Autodesk Inventor part; units mm, degrees
ref_plane "YZ Plane" through (0, 0, 0) normal (1, 0, 0) x (0, 1, 0)
ref_plane "XZ Plane" through (0, 0, 0) normal (0, 1, 0) x (-1, 0, 0)
ref_plane "XY Plane" through (0, 0, 0) normal (0, 0, 1) x (1, 0, 0)
sketch "Sketch1" plane through (0, 0, 0) normal (0, 1, 0) x (-1, 0, 0)
  line L0 (29, 0) -> (29, -12)
  line L1 (27, -14) -> (16, -14)
  line L2 (-16, -14) -> (-27, -14)
  line L3 (-29, -12) -> (-29, 12)
  line L4 (-27, 14) -> (-16, 14)
  line L5 (16, 14) -> (27, 14)
  line L6 (29, 12) -> (29, 0)
  line L7 (14, -16) -> (14, -40)
  line L8 (12, -42) -> (-12, -42)
  line L9 (-14, -40) -> (-14, -16)
  line L10 (-14, 16) -> (-14, 40)
  line L11 (-12, 42) -> (12, 42)
  line L12 (14, 40) -> (14, 16)
  arc A0 (29, 12) -> (27, 14) centre (27, 12) ccw
  arc A1 (27, -14) -> (29, -12) centre (27, -12) ccw
  arc A2 (16, -14) -> (14, -16) centre (16, -16) ccw
  arc A3 (12, -42) -> (14, -40) centre (12, -40) ccw
  arc A4 (-14, -40) -> (-12, -42) centre (-12, -40) ccw
  arc A5 (-14, -16) -> (-16, -14) centre (-16, -16) ccw
  arc A6 (-29, -12) -> (-27, -14) centre (-27, -12) ccw
  arc A7 (-27, 14) -> (-29, 12) centre (-27, 12) ccw
  arc A8 (-16, 14) -> (-14, 16) centre (-16, 16) ccw
  arc A9 (-12, 42) -> (-14, 40) centre (-12, 40) ccw
  arc A10 (14, 40) -> (12, 42) centre (12, 40) ccw
  arc A11 (14, 16) -> (16, 14) centre (16, 16) ccw
  point P0 (0, 0)
  point P1 (29, -14)
  point P2 (14, -14)
  point P3 (-14, -14)
  point P4 (-29, -14)
  point P5 (-29, 14)
  point P6 (-14, 14)
  point P7 (14, -42)
  point P8 (-14, 42)
  point P9 (14, 42)
  dimension "d2" = 14
  dimension "d4" = 15
  dimension "d5" = 28
  dimension "d7" = 28
  dimension "d8" = 28
  dimension "d12" = 2
extrude "Extrusion1" add sketch "Sketch1" along normal blind 1
sketch "Sketch2" plane through (0, 1, 0) normal (0, 1, 0) x (1, 0, 0)
  circle A0 centre (0, 0) radius 19
  dimension "d15" = 38
extrude "Extrusion2" add sketch "Sketch2" along normal blind 10
sketch "Sketch3" plane through (0, 11, 0) normal (0, 1, 0) x (1, 0, 0)
  circle A0 centre (0, 0) radius 8
  dimension "d18" = 16
extrude "Extrusion3" add sketch "Sketch3" along normal blind 7
sketch "Sketch4" plane through (0, 18, 0) normal (0, 1, 0) x (1, 0, 0)
  circle A0 centre (0, 0) radius 13.5
  dimension "d21" = 27
extrude "Extrusion4" add sketch "Sketch4" along normal blind 40
sketch "Sketch5" plane through (0, 58, 0) normal (0, 1, 0) x (1, 0, 0)
  line L0 (0, 41.9572) -> (12, 41.9572)
  line L1 (14, 39.9572) -> (14, -40)
  line L2 (12, -42) -> (-12, -42)
  line L3 (-14, -40) -> (-14, 39.9572)
  line L4 (-12, 41.9572) -> (0, 41.9572)
  arc A0 (-12, 41.9572) -> (-14, 39.9572) centre (-12, 39.9572) ccw
  arc A1 (14, 39.9572) -> (12, 41.9572) centre (12, 39.9572) ccw
  arc A2 (12, -42) -> (14, -40) centre (12, -40) ccw
  arc A3 (-14, -40) -> (-12, -42) centre (-12, -40) ccw
  point P0 (0, 0)
  point P1 (-14, 41.9572)
  dimension "d24" = 2
extrude "Extrusion5" add sketch "Sketch5" along normal blind 1
sketch "Sketch6" plane through (0, 1, 0) normal (0, 1, 0) x (1, 0, 0)
  line L0 (0, 0) -> (0, 36)
  line L1 (0, 0) -> (0, -36)
  circle A0 centre (0, 36) radius 2.5
  circle A1 centre (0, -36) radius 2.5
  dimension "d27" = 36
  dimension "d28" = 36
  dimension "d29" = 5
  dimension "d30" = 5
extrude "Extrusion6" add sketch "Sketch6" along normal blind 58
sketch "Sketch7" plane through (0, 0, 0) normal (0, -1, 0) x (1, 0, 0)
  circle A0 centre (0, 0) radius 15
  dimension "d33" = 30
extrude "Extrusion7" add sketch "Sketch7" along normal blind 32
sketch "Sketch8" plane through (0, -32, 0) normal (0, -1, 0) x (1, 0, 0)
  circle A0 centre (0, 0) radius 8
  dimension "d36" = 16
extrude "Extrusion8" add sketch "Sketch8" along normal blind 43
fillet "Fillet1" radius 5 1 edges at (-15, -32, 0)
sketch "Sketch9" plane through (0, -75, 0) normal (0, -1, 0) x (1, 0, 0)
  circle A0 centre (0, 0) radius 4
  circle A1 centre (0, 0) radius 12.3979
  dimension "d40" = 8
extrude "Extrusion9" cut sketch "Sketch9" against normal blind 20
fillet "Fillet2" radius 5 1 edges at (-4, -55, 0)
sketch "Sketch10" plane through (14, 0, 40) normal (1, 0, 0) x (0, 0, -1)
  line L0 (36, -75) -> (44, -75)
  line L1 (36, -75) -> (38.5, -75)
  line L2 (38.5, -75) -> (38.5, -71.9713)
  line L3 (38.5, -71.9713) -> (36, -71.9713)
  line L4 (36, -71.9713) -> (36, -75)
  line L5 (44, -59.899) -> (44, -75)
  line L6 (44, -75) -> (41.5, -75)
  line L7 (41.5, -75) -> (41.5, -71.9713)
  line L8 (41.5, -71.9713) -> (44, -71.9713)
  line L9 (44, -71.9713) -> (44, -75)
  point P0 (40, 0)
  dimension "d44" = 2.5
  dimension "d45" = 2.5
extrude "Extrusion10" cut sketch "Sketch10" against normal blind 20
sketch "Sketch11" plane through (-3.7081, -71.9713, 1.5) normal (0, 0, 1) x (1, 0, 0)
  line L0 (7.4162, -3.0287) -> (0, -3.0287)
  line L1 (3.7081, -3.0287) -> (8.9248, -1.5011)
  line L2 (8.9248, -1.5011) -> (8.9248, -4.1511)
  line L3 (8.9248, -4.1511) -> (-1.9974, -3.8292)
  line L4 (-1.9974, -3.8292) -> (-1.4278, -1.5011)
  line L5 (-1.4278, -1.5011) -> (3.7081, -3.0287)
  point P0 (3.7081, 71.9713)
extrude "Extrusion11" cut sketch "Sketch11" against normal blind 20
sketch "Sketch12" plane through (0, 59, 0) normal (0, 1, 0) x (1, 0, 0)
  circle A0 centre (0, 20) radius 3
  circle A1 centre (0, -20) radius 3
  point P0 (0, 0)
  dimension "d51" = 6
  dimension "d52" = 6
extrude "Extrusion12" cut sketch "Sketch12" against normal blind 20
properties part number "marcadorNUEVO"
Could you check a few things on this model? Use its own coordinates, in mm. A direction names the side the tool comes from. Give positions to 0.01 mm unless a question says otherwise; leave off trailing zeros. Loops run counter-clockwise (first coordinate to the right, second up) from the corner with the lowest first, then second, coordinate; pieces in that order, holes last. Notation, with made-up numbers: M 86.25,-10.5 L 140.25,-10.5 A17 ccw 140.25,12.5 Z; hole C -26.75,5 d3. An arc over 180 degrees is marked long. Answer as a JSON object with one key per item and string values.
Q1. Suppose I cut it at B-B, the plane y = 47. List the corners of the cut face in (x, z) for me, plus the area to 3 significant figures.
Values found:
{"outline": "C 0,0 d27; C 0,-36 d5; C 0,36 d5", "area": "612 mm²"}
Q2. If we mould it in two halves opening along Z, with no side actions, what happens to faces 1 (the flat face through (13, 0, 10)), 2 (the cylindrical face through (-14.985, -13.311, -0.66)), 3 (the cylindrical face through (-0.54, 29.1, 33.56))? For each: pulls with the +Z half, pulls with the -Z half, needs draft (parallel to the pull), parting line crosses it, or undercut.
Values found:
{"face 1": "needs draft", "face 2": "parting line crosses it", "face 3": "undercut"}
Q3. Suppose I cut it at D-D, the plane y = -3. List the corners of the cut face in (x, z) for me, plus the area to 3 significant figures.
Values found:
{"outline": "C 0,0 d30", "area": "707 mm²"}
Q4. Suppose I cut it at A-A, the plane z = 24.5. List the corners of the cut face in (x, y) for me.
Values found:
{"outline": "M -14,0 L 14,0 L 14,1 L -14,1 Z; M -14,58 L 14,58 L 14,59 L -14,59 Z"}
Q5. For faces 4 (the flat face through (0, -73, 1.5)), 5 (the cylindrical face through (-0.65, 58.51, -17.07)), 6 (the flat face through (0, -73, -1.5)), 7 (the cylindrical face through (-0.521, -67.005, 3.966)), 8 (the flat face through (-0.3, 11, 8.2)), which set-ups out of +Z, -Z, +X, -X, +Y, -Y let a thin tool reach every point of the face, with its end or its side?
Values found:
{"face 4": "+Z, +X, -X, -Y", "face 5": "+Y", "face 6": "-Z, +X, -X, -Y", "face 7": "-Y", "face 8": "none"}
Q6. Suppose I cut it at C-C, the plane z = 36. List the corners of the cut face in (x, y) for me.
Values found:
{"outline": "M -14,0 L 14,0 L 14,1 L 2.5,1 L 2.5,58 L 14,58 L 14,59 L -14,59 L -14,58 L -2.5,58 L -2.5,1 L -14,1 Z"}
Q7. For P1, Ø4, axis at x = -8, y = -50.5, coming from the +Z side; P2, Ø0.5, axis at x = 21, y = 0.5, coming from the +Z side; P3, Ø1.3, axis at x = -1.5, z = 2, coming from the -Y side, each with a flat end and sliding along its axis, tell me the tip position at first contact or that it passes through.
Values found:
{"P1": "stops at z = 5.29", "P2": "stops at z = 14", "P3": "stops at y = -74.68"}
Q8. If I drill on probe 1 along Z at (x, y) = (0, 58.7); probe 2 along Y at (x, z) = (-8, 1); probe 3 along X at (y, z) = (58.7, 20), over which ranges is the centre line in solid material (lowest first)? Write a range as [from, to].
Values found:
{"probe 1": "z = [-41.96, -23], [-17, 17], [23, 42]", "probe 2": "y = [-32, 11], [18, 59]", "probe 3": "x = [-14, -3], [3, 14]"}
